The listing builds one solid part. Answer for the finished solid, in the listing's coordinates (mm). A direction names the side the tool comes from. Round coordinates to 2 decimals unless told otherwise and drop trailing zeros. Write each loop counter-clockwise with the first axis right and the second up, starting at its lowest first coordinate (ties: lowest second). Pieces come first, ordered by that corner, then holes. Notation, with made-up numbers: (23.25, 72) -> (63.25, 72) arc R25 cw to (63.25, 111) -> close; hole circle Ø1 at (-9, 14.25). An arc over 180 degrees is marked (long way). Write each question's results on one line, items separated by ' | '. Start each with the question number.
```python
from build123d import *

# Parameters (mm, degrees)
SKETCH1_W      = 20
SKETCH1_H      = 20
EXTRUDE1_DEPTH = 40


with BuildPart() as part:
    # Sketch1 → Extrude1 (new body)
    with BuildSketch(Plane.XY):
        Polygon((0, 140), (100, 140), (100, 100), (65, 100), (54.5, 70), (65, 40), (100, 40), (100, 0), (0, 0), (0, 20), (-20, 20), (-20, 40), (-40, 40), (-40, 100), (-20, 100), (-20, 120), (0, 120), align=None)
        with Locations((30, 110)):
            Rectangle(SKETCH1_W, SKETCH1_H, mode=Mode.SUBTRACT)
    extrude(amount=EXTRUDE1_DEPTH)


solid = part.part
```
Q1. Each of these flat-tipped pins is pushed along its axis until it touches: pin 1 (8 mm diameter, centred on x = -19.5, z = 23.5, fed in from -Y); pin 2 (3 mm diameter, centred on y = 41, z = 21.5, fed in from +X); pin 3 (16 mm diameter, centred on x = -26, z = 11, fed in from +Y); pin 4 (4 mm diameter, centred on y = 45.5, z = 18.5, fed in from +X) (3 decimals). Where does it stop, or does it pass through?
Q2. Determine the mould class of faces 5 (the flat face through (100, 120, 20)), 6 (the flat face through (-30, 100, 20)), 7 (the flat face through (82, 40, 20)) for opening direction Y: pulls with the +Y half, pulls with the -Y half, needs draft (parallel to the pull), parting line crosses it, or undercut.
Q3. For faces 1 (the flat face through (30, 120, 20)), 2 (the flat face through (0, 10, 20)), 3 (the flat face through (-10, 120, 20)), 4 (the flat face through (59.823, 85.21, 19.72)), determine the directions among +Z, -Z, +X, -X, +Y, -Y from which every point of the face is accessible in a straight line to the end or side of a thin tool.
Q4. The part is cut by section D-D, the plane x = 81. Write down the section's boundary in (y, z), then the cut area to 3 significant figures.
Q5. Find the intervals of material crossed by line 1 (X direction, y = 103, z = 22.5); line 2 (Y direction, x = 88.5, z = 2.5); line 3 (Y direction, x = 25.5, z = 5), in increasing order.
Q6. The part is cut by section C-C, the plane y = 16. Write down the section's boundary in (x, z).
Q7. The part is cut by section A-A, the plane x = 34. Write down the section's boundary in (y, z).
Q8. The part is cut by section B-B, the plane z = 14. Write down the section's boundary in (x, y), then the cut area to 3 significant figures.
Answers follow:
1) pin 1: y = 20 | pin 2: x = 100 | pin 3: y = 120 | pin 4: x = 63.775
2) face 5: needs draft | face 6: pulls with the +Y half | face 7: undercut
3) face 1: +Z, -Z | face 2: +Z, -Z, -X, -Y | face 3: +Z, -Z, -X, +Y | face 4: +Z, -Z, +X
4) outline: (0, 0) -> (40, 0) -> (40, 40) -> (0, 40) -> close; (100, 0) -> (140, 0) -> (140, 40) -> (100, 40) -> close | area: 3,200 mm^2
5) line 1: -20 to 20, 40 to 100 | line 2: 0 to 40, 100 to 140 | line 3: 0 to 100, 120 to 140
6) outline: (0, 0) -> (100, 0) -> (100, 40) -> (0, 40) -> close
7) outline: (0, 0) -> (100, 0) -> (100, 40) -> (0, 40) -> close; (120, 0) -> (140, 0) -> (140, 40) -> (120, 40) -> close
8) outline: (-40, 40) -> (-20, 40) -> (-20, 20) -> (0, 20) -> (0, 0) -> (100, 0) -> (100, 40) -> (65, 40) -> (54.5, 70) -> (65, 100) -> (100, 100) -> (100, 140) -> (0, 140) -> (0, 120) -> (-20, 120) -> (-20, 100) -> (-40, 100) -> close; hole (20, 100) -> (40, 100) -> (40, 120) -> (20, 120) -> close | area: 14,400 mm^2
